Autodesk Inventor part; units mm, degrees
ref_plane "YZ Plane" through (0, 0, 0) normal (1, 0, 0) x (0, 1, 0)
ref_plane "XZ Plane" through (0, 0, 0) normal (0, 1, 0) x (-1, 0, 0)
ref_plane "XY Plane" through (0, 0, 0) normal (0, 0, 1) x (1, 0, 0)
sketch "Sketch1" plane through (0, 0, 0) normal (0, 1, 0) x (-1, 0, 0)
  line L0 (0, 0) -> (10, 0)
  line L1 (5, 0) -> (5, -10)
  line L2 (10, -10) -> (0, -10)
  line L3 (5, -5) -> (7.5, -5)
  line L4 (7.5, -5) -> (10, 0)
  line L5 (7.5, -5) -> (10, -10)
  line L6 (5, -5) -> (2.5, -5)
  line L7 (2.5, -5) -> (0, -10)
  line L8 (2.5, -5) -> (0, 0)
  line L9 (5, 0) -> (9.5, 0)
  line L10 (9.5, 0) -> (7.5, -5)
  line L11 (5, 0) -> (0.5, 0)
  line L12 (0.5, 0) -> (2.5, -5)
  line L13 (2.5, -5) -> (0.5, -10)
  line L14 (7.5, -5) -> (9.5, -10)
  dimension "d0" = 10
  dimension "d1" = 10
  dimension "d2" = 2.5
  dimension "d3" = 2.5
  dimension "d4" = 4.5
  dimension "d5" = 4.5
extrude "Extrusion1" add sketch "Sketch1" along normal blind 5 contours L0 L1 L6 L12 | L6 L1 L2 L13 | L0 L10 L3 L1 | L3 L14 L2 L1
properties part number "dishConnector_3DPrint"
Check sheet for the modelled part. Datum: model origin and axes. Units: mm. A direction names the side the tool comes from. Give positions to 0.01 mm unless a question says otherwise; leave off trailing zeros. Loops run counter-clockwise (first coordinate to the right, second up) from the corner with the lowest first, then second, coordinate; pieces in that order, holes last. Notation, with made-up numbers: M 77,-29 L 132,-29 A18 cw 132,-21 Z; hole C 3,79.5 d7. An arc over 180 degrees is marked long. Use a Markdown table: item, result. Add a question column.
Q1. Sectioned sample at C-C, the plane x = -7.75. Record the cut outline in (y, z) (3 decimals).
Q2. Sectioned sample at B-B, the plane y = 2.7. Record the cut outline in (x, z).
Q3. Tool access check on faces 1 (the flat face through (-1.5, 2.5, -2.5)), 2 (the flat face through (-5, 0, -5)), 3 (the flat face through (-8.5, 2.5, -2.5)). Record the directions out of +Z, -Z, +X, -X, +Y, -Y that give a thin tool (end or side, any length) a straight path to the whole face; none if there is none.
Q4. Sectioned sample at D-D, the plane z = -5.75. Record the cut outline in (x, y), then the cut area to 3 significant figures.
Q5. Go/stop test with flat-tipped pins: pin 1 (1 mm diameter, centred on y = 3.5, z = -2, fed in from +X); pin 2 (1.5 mm diameter, centred on y = 2.5, z = -1.5, fed in from -X). Record where each tip stops, or that it passes through.
Q6. Sectioned sample at A-A, the plane x = -1.5. Record the cut outline in (y, z), then the cut area to 3 significant figures.
Q7. Mould release check, pull along Z, two halves, no side actions. Record for faces 4 (the flat face through (-5, 5, -5)), 5 (the flat face through (-8.5, 2.5, -7.5)), 6 (the flat face through (-5, 2, -10)), 7 (the flat face through (-5, 2, 0)): pulls with the +Z half, pulls with the -Z half, needs draft (parallel to the pull), parting line crosses it, or undercut.
Q8. Scan lines: line 1 along X through (y, z) = (0.9, -3); line 2 along X through (y, z) = (4.05, -4.25). Record each from-to range of solid material in increasing order. Write a range as [from, to].
Verdict:
| question | item | result |
|---|---|---|
| 1 | outline | M 0,-10 L 5,-10 L 5,-5.625 L 0,-5.625 Z; M 0,-4.375 L 5,-4.375 L 5,0 L 0,0 Z |
| 2 | outline | M -9.5,-10 L -0.5,-10 L -2.5,-5 L -0.5,0 L -9.5,0 L -7.5,-5 Z |
| 3 | face 1 | +X, +Y, -Y |
| 3 | face 2 | +Z, -Z, +X, -X, -Y |
| 3 | face 3 | -X, +Y, -Y |
| 4 | outline | M -7.8,0 L -2.2,0 L -2.2,5 L -7.8,5 Z |
| 4 | area | 28.0 mm^2 |
| 5 | pin 1 | x = -1.1 |
| 5 | pin 2 | x = -9.2 |
| 6 | outline | M 0,-10 L 5,-10 L 5,-7.5 L 0,-7.5 Z; M 0,-2.5 L 5,-2.5 L 5,0 L 0,0 Z |
| 6 | area | 25.0 mm^2 |
| 7 | face 4 | needs draft |
| 7 | face 5 | undercut |
| 7 | face 6 | pulls with the -Z half |
| 7 | face 7 | pulls with the +Z half |
| 8 | line 1 | [-8.3, -1.7] |
| 8 | line 2 | [-7.8, -2.2] |
